Design review of the part built by this model. Coordinates are the model's own, in mm. A direction names the side the tool comes from. Round coordinates to 2 decimals unless told otherwise and drop trailing zeros. Order: outer loops, then holes, each group sorted by start corner. A loop starts at its lowest first (then second) coordinate and runs counter-clockwise, first axis right, second up. Notation, with made-up numbers: M 14.5,31 L 71.5,31 A13 cw 71.5,36 Z; hole C 14,-38.5 d7. An arc over 180 degrees is marked long. Use a Markdown table: item, result. Add a question column.
(1) Machinability: for faces 5 (the face through (-41, 9, 9)), 6 (the face through (29, -13.43, 8.98)), 7 (the face through (-54.5, 0.3, -16.3)), 8 (the face through (3, 0, -6)), which of the approach directions +Z, -Z, +X, -X, +Y, -Y give a long, thin tool a straight path to every point of the face, cutting with its end or side? Answer none if there is none.
(2) To check wall thickness, follow probe 1 along Y at (x, z) = (-28, 0); probe 2 along X at (y, z) = (-14, -12). State the ranges of each line that lie inside material, in increasing order. Write a range as from..to.
(3) For pin 1 (20.5 mm diameter, centred on y = -1.5, z = -8, fed in from -X); pin 2 (15 mm diameter, centred on y = 0.5, z = -7, fed in from -X); pin 3 (4 mm diameter, centred on x = -16, z = -14.5, fed in from +Y), all flat-tipped, find the tip position at first contact; note any pin that passes through.
(4) The part is to be moulded in two halves that separate along Y. For faces 1 (the face through (32, 0, -7)), 2 (the face through (-44, 8, -10)), 3 (the face through (30.48, 15.62, -3.47)), 4 (the face through (-34, 9, -9)), say which applies: released by +Y, released by -Y, zero draft, split by the parting line, or undercut.
(5) Take a section at A-A (x = -8). Write out the cut boundary in (y, z), then the cut area to 3 significant figures.
```python
from build123d import *

# Parameters (mm, degrees)
F2_R        = 6
F1_FACE_R   = 25
F1_FACE_R_2 = 16
F3_DEPTH    = 1.5


with BuildPart() as f1:
    # F0 (on Front) → F1 (revolve)
    with BuildSketch(Plane.XZ):
        with BuildLine():
            Line((-26, 6), (32, 6))
            Line((32, 6), (32, 16))
            Line((32, 16), (29, 16))
            Line((29, 16), (29, 20))
            Line((29, 20), (12, 20))
            Line((12, 20), (12, 31))
            Line((12, 31), (0, 31))
            ThreePointArc((0, 31), (-6, 25), (-12, 31))
            Line((-12, 31), (-56, 31))
            Line((-56, 31), (-56, 16))
            Line((-56, 16), (-44, 16))
            Line((-44, 16), (-44, 12.5))
            Line((-44, 12.5), (-41, 12.5))
            Line((-41, 12.5), (-41, 20.5))
            Line((-41, 20.5), (-34, 20.5))
            Line((-34, 20.5), (-34, 12.5))
            Line((-34, 12.5), (-26, 12.5))
            Line((-26, 12.5), (-26, 6))
        make_face()
    revolve(axis=Axis((0, 0, 0), (1, 0, 0)))

    # F2
    f2_edges = [f1.edges().sort_by_distance(p)[0] for p in [
        (-56, 0, -31),
    ]]
    fillet(f2_edges, radius=F2_R)

    # F1_face (on face) → F3 (cut)
    with BuildSketch(Plane(origin=(-56, 0, 0), x_dir=(0, -1, 0), z_dir=(-1, 0, 0))):
        Circle(F1_FACE_R)
        Circle(F1_FACE_R_2, mode=Mode.SUBTRACT)
    extrude(amount=-F3_DEPTH, mode=Mode.SUBTRACT)


solid = f1.part
```
Verdict:
| question | item | result |
|---|---|---|
| 1 | face 5 | none |
| 1 | face 6 | +X |
| 1 | face 7 | -X |
| 1 | face 8 | +X, -X |
| 2 | probe 1 | y = -31..-12.5, 12.5..31 |
| 2 | probe 2 | x = -54.5..-41, -34..29 |
| 3 | pin 1 | stops at x = -54.5 |
| 3 | pin 2 | stops at x = -44 |
| 3 | pin 3 | stops at y = 28.37 |
| 4 | face 1 | zero draft |
| 4 | face 2 | undercut |
| 4 | face 3 | split by the parting line |
| 4 | face 4 | undercut |
| 5 | outline | C 0,0 d50.69; hole C 0,0 d12 |
| 5 | area | 1,900 mm^2 |
